Build history of the part. All positions in model axes, mm. A direction names the side the tool comes from. Round coordinates to 2 decimals unless told otherwise and drop trailing zeros. Write each loop counter-clockwise with the first axis right and the second up, starting at its lowest first coordinate (ties: lowest second). Pieces come first, ordered by that corner, then holes. Notation, with made-up numbers: (13, 89.5) - (23, 89.5) arc R31 ccw to (23, 114.5) - close; hole circle Ø1 at (-35, 68). An arc over 180 degrees is marked (long way). One line per question, with ' | ' between items.
from build123d import *

# Parameters (mm, degrees)
BOSS_EXTRUDE1_START     = -2.5
BOSS_EXTRUDE1_OUTLINE_R = 2.075
BOSS_EXTRUDE1_DEPTH     = 5
FILLET1_R               = 10
FILLET2_R               = 2
SKETCH6_R               = 2.6
CUT_EXTRUDE3_DEPTH      = 0.6
CUT_EXTRUDE4_START      = -0.6
SKETCH7_R               = 2.6
CUT_EXTRUDE4_DEPTH      = 0.6


# Read off the part's stored shape, not the designer's step: Boss-Extrude1
with BuildPart() as part:
    # Boss-Extrude1 outline → Boss-Extrude1 (new body)
    with BuildSketch(Plane(origin=(0, 0, 0), x_dir=(0, 0, -1), z_dir=(1, 0, 0)).offset(BOSS_EXTRUDE1_START)):
        with BuildLine():
            add(Edge.make_bspline(
                [(-11.467537503, 5.350641642), (-9.989640807, 4.583198508), (-7.178473446, 3.56515844), (-2.794711607, 2.423489001), (1.31753402, 1.289926051), (5.278860449, -0.285822235), (9.053028754, -1.966642772), (11.935810136, -3.144477132), (13.583881592, -3.694358455), (13.981041238, -3.818362685)],
                knots=[0.086674, 0.086674, 0.086674, 0.086674, 0.25, 0.375, 0.5, 0.625, 0.75, 0.875, 0.914505017, 0.914505017, 0.914505017, 0.914505017], degree=3))
            ThreePointArc((-11.467537503, 5.350641642), (-17.181514848, 7.27580405), (-12.959070193, 2.971533086))
            add(Edge.make_bspline(
                [(-12.959070193, 2.971533086), (-12.497149124, 2.725216721), (-10.724559711, 1.865083664), (-7.538415314, 0.763759759), (-3.469271241, -0.293699416), (0.432825124, -1.371499483), (4.151444935, -2.850197037), (7.925726422, -4.529354156), (10.977952232, -5.779484012), (12.799789723, -6.384662727), (13.276371809, -6.531370761)],
                knots=[0.080415635, 0.080415635, 0.080415635, 0.080415635, 0.125, 0.25, 0.375, 0.5, 0.625, 0.75, 0.875, 0.9184538, 0.9184538, 0.9184538, 0.9184538], degree=3))
            ThreePointArc((13.276371809, -6.531370761), (19.30544163, -6.649326649), (13.981041238, -3.818362685))
        make_face()
        with Locations((16.305, -5.87)):
            Circle(BOSS_EXTRUDE1_OUTLINE_R, mode=Mode.SUBTRACT)
        with Locations((-14.555, 5.629165125)):
            Circle(BOSS_EXTRUDE1_OUTLINE_R, mode=Mode.SUBTRACT)
    extrude(amount=BOSS_EXTRUDE1_DEPTH)

    # Fillet1
    fillet1_edges = [part.edges().sort_by_distance(p)[0] for p in [
        (0, -6.531370761, -13.276371809),
        (0, 5.350641642, 11.467537503),
    ]]
    fillet(fillet1_edges, radius=FILLET1_R)

    # Fillet2
    fillet2_edges = [part.edges().sort_by_distance(p)[0] for p in [
        (0, -3.818362685, -13.981041238),
        (0, 2.971533086, 12.959070193),
    ]]
    fillet(fillet2_edges, radius=FILLET2_R)

    # Sketch6 → Cut-Extrude3 (cut)
    with BuildSketch(Plane(origin=(2.5, 0, 0), x_dir=(0, 0, -1), z_dir=(1, 0, 0))):
        with Locations((-14.555, 5.629165125)):
            Circle(SKETCH6_R)
        with Locations((16.305, -5.87)):
            Circle(SKETCH6_R)
    extrude(amount=-CUT_EXTRUDE3_DEPTH, mode=Mode.SUBTRACT)

    # Sketch7 → Cut-Extrude4 (cut)
    with BuildSketch(Plane.ZY.offset(2.5).offset(CUT_EXTRUDE4_START)):
        with Locations(Location((14.555, 5.629165125, 0), (0, 0, 180))):
            Circle(SKETCH7_R)
        with Locations(Location((-16.305, -5.87, 0), (0, 0, 180))):
            Circle(SKETCH7_R)
    extrude(amount=CUT_EXTRUDE4_DEPTH, mode=Mode.SUBTRACT)


solid = part.part
Q1. Drop flat-ended pins along their axis: pin 1 (2 mm diameter, centred on x = 0, z = 12, fed in from +Y); pin 2 (2.5 mm diameter, centred on y = -5.5, z = -16, fed in from -X); pin 3 (1 mm diameter, centred on x = -1.5, y = -6.5, fed in from -Z); pin 4 (1.5 mm diameter, centred on x = 0.5, z = 11.5, fed in from +Y). Give the stop position or say it passes through.
Found:
pin 1: y = 8.31 | pin 2: through | pin 3: z = -19.4 | pin 4: y = 7.7
Q2. Saw through at B-B, the plane x = 0.45. State how many separate pieces and enclosed holes the cut face has, then the cut area to 3 significant figures.
Found:
separate pieces: 1 | enclosed holes: 2 | area: 112 mm^2
Q3. Which spindle directions (+Z, -Z, +X, -X, +Y, -Y) get a long thin tool onto all of the face, cutting with end or side? Do faces 4 (the cylindrical face through (2.204, -5.089, -18.785)), 5 (the cylindrical face through (-2.196, 5.515, 17.152)), 6 (the cylindrical face through (-0.035, 6.729, 17.453)). Say none if no direction does.
Found:
face 4: +X | face 5: -X | face 6: +X, -X
Q4. Saw through at A-A, the plane z = -15.5. List the corners of the cut face in (x, y).
Found:
outline: (-2.5, -8.86) - (2.5, -8.86) - (2.5, -8.34) - (1.9, -8.34) - (1.9, -7.78) - (-1.9, -7.78) - (-1.9, -8.34) - (-2.5, -8.34) - close; (-2.5, -3.4) - (-1.9, -3.4) - (-1.9, -3.96) - (1.9, -3.96) - (1.9, -3.4) - (2.5, -3.4) - (2.5, -2.88) - (-2.5, -2.88) - close
Q5. Drill centre lines: L1, parallel to Y at x = 0.6, z = 15; L2, parallel to Z at x = 0.7, y = 4.75; L3, parallel to Y at x = -1.55, z = 15.5. Where is each one in solid material? Low to high. Write a range as from..to.
Found:
L1: 2.56..3.6, 7.66..8.7 | L2: 9.34..12.68, 16.43..17.53 | L3: 2.68..3.78, 7.48..8.58
Q6. Pull direction Y, two halves, no side cores. Call faces 1 (the flat face through (-1.9, -4, -15)), 2 (the cylindrical face through (-0.035, -6.352, -19.367)), 3 (the flat face through (-2.5, 0, -1)): +Y half, -Y half, draft (parallel to the pull), parting line (faces both ways), or undercut.
Found:
face 1: undercut | face 2: parting line | face 3: draft
